from build123d import *

# Parameters (mm, degrees)
SKETCH1_W           = 12
SKETCH1_H           = 64.5
BOSS_EXTRUDE1_DEPTH = 5
FILLET1_R           = 6
SKETCH2_R           = 2
CUT_EXTRUDE1_DEPTH  = 34.182261828
BOSS_EXTRUDE2_START = 5
SKETCH3_R           = 6
SKETCH3_R_2         = 2
BOSS_EXTRUDE2_DEPTH = 5
SKETCH4_R           = 2
CUT_EXTRUDE2_DEPTH  = 34.182261828
CUT_EXTRUDE3_DEPTH  = 2.5


with BuildPart() as part:
    # Sketch1 → Boss-Extrude1 (new body)
    with BuildSketch(Plane(origin=(0, 0, 0), x_dir=(1, 0, 0), z_dir=(0, 1, 0))):
        Rectangle(SKETCH1_W, SKETCH1_H)
    extrude(amount=BOSS_EXTRUDE1_DEPTH)

    # Fillet1
    fillet1_edges = [part.edges().sort_by_distance(p)[0] for p in [
        (-6, 2.5, -32.25),
        (6, 2.5, -32.25),
        (-6, 2.5, 32.25),
        (6, 2.5, 32.25),
    ]]
    fillet(fillet1_edges, radius=FILLET1_R - 0.0001)  # a hair under: the kernel refuses the full size

    # Sketch2 → Cut-Extrude1 (cut, through all)
    with BuildSketch(Plane(origin=(0, 5, 0), x_dir=(1, 0, 0), z_dir=(0, 1, 0))):
        with Locations(Location((0, -26.25, 0), (0, 0, 270))):
            Circle(SKETCH2_R)
        with Locations(Location((0, 26.25, 0), (0, 0, 270))):
            Circle(SKETCH2_R)
    extrude(amount=-CUT_EXTRUDE1_DEPTH, mode=Mode.SUBTRACT)

    # Sketch3 → Boss-Extrude2 (add)
    # profile 1 of 2: a face of its own
    with BuildSketch(Plane(origin=(0, 5, 0), x_dir=(1, 0, 0), z_dir=(0, 1, 0)).offset(BOSS_EXTRUDE2_START)):
        with Locations(Location((0, -26.25, 0), (0, 0, 270))):
            Circle(SKETCH3_R)
        with Locations(Location((0, -26.25, 0), (0, 0, 270))):
            Circle(SKETCH3_R_2, mode=Mode.SUBTRACT)
    # profile 2 of 2: a face of its own
    with BuildSketch(Plane(origin=(0, 5, 0), x_dir=(1, 0, 0), z_dir=(0, 1, 0)).offset(BOSS_EXTRUDE2_START)):
        with Locations(Location((0, 26.25, 0), (0, 0, 90))):
            Circle(SKETCH3_R)
        with Locations(Location((0, 26.25, 0), (0, 0, 270))):
            Circle(SKETCH3_R_2, mode=Mode.SUBTRACT)
    extrude(amount=-BOSS_EXTRUDE2_DEPTH)

    # Sketch4 → Cut-Extrude2 (cut, through all)
    with BuildSketch(Plane(origin=(0, 5, 0), x_dir=(1, 0, 0), z_dir=(0, 1, 0))):
        with Locations(Location((0, 15, 0), (0, 0, 270))):
            Circle(SKETCH4_R)
        with Locations(Location((0, -15, 0), (0, 0, 270))):
            Circle(SKETCH4_R)
    extrude(amount=-CUT_EXTRUDE2_DEPTH, mode=Mode.SUBTRACT)

    # Sketch5 → Cut-Extrude3 (cut)
    with BuildSketch(Plane.XZ):
        Polygon((4.618802154, 26.25), (2.309401077, 30.25), (-2.309401077, 30.25), (-4.618802154, 26.25), (-2.309401077, 22.25), (2.309401077, 22.25), align=None)
        Polygon((2.309401077, -22.25), (-2.309401077, -22.25), (-4.618802154, -26.25), (-2.309401077, -30.25), (2.309401077, -30.25), (4.618802154, -26.25), align=None)
    extrude(amount=-CUT_EXTRUDE3_DEPTH, mode=Mode.SUBTRACT)


solid = part.part
For this review, take the finished solid that the model builds, in its own axes (mm). A direction names the side the tool comes from. Give positions to 0.01 mm unless a question says otherwise; leave off trailing zeros. Order: outer loops, then holes, each group sorted by start corner. A loop starts at its lowest first (then second) coordinate and runs counter-clockwise, first axis right, second up. Notation, with made-up numbers: M 65.5,57.25 L 92.5,57.25 A17 ccw 92.5,74.25 Z; hole C -4,78 d9. An arc over 180 degrees is marked long. Answer in a Markdown table with one row per item. Add a question column.
(1) Consider section C-C on y = 7.5. State the section outline as (x, z) points.
(2) For faces 5 (the face through (0, 1, 22.25)), 6 (the face through (-0.264, 7.535, -20.256)), 7 (the face through (0, 10, 29)), list the 3-axis set-ups (+Z, -Z, +X, -X, +Y, -Y) from which the entire face can be reached by the end or side of a thin tool; tool diameter is ignored.
(3) Consider section A-A on z = -15. State the section outline as (x, y) points.
(4) Consider section B-B on x = -1.25. Give the number of separate pieces and of enclosed holes in the cut face, and give its area (3 significant figures).
(5) Consider section D-D on z = -7.5. State the section outline as (x, y) points.
(6) For pin 1 (3 mm diameter, centred on x = 1, z = 2, fed in from +Y); pin 2 (2.5 mm diameter, centred on x = -1.5, z = -27.5, fed in from -Y); pin 3 (3.5 mm diameter, centred on x = 0, z = -15, fed in from +Y); pin 4 (6 mm diameter, centred on x = 4.5, y = 7.5, fed in from -Z), all flat-tipped, find the tip position at first contact; note any pin that passes through.
(7) Wall thickness on probe 1 along Z at (x, y) = (1.75, 7.25); probe 2 along X at (y, z) = (1, 15); probe 3 along X at (y, z) = (9.5, 28): over which ranges is each line inside the solid? List them lowest first. Write a range as [from, to].
(8) Mouldability with a two-part tool opening along Z and no side actions: class faces 1 (the face through (-4.289, 2.535, -30.446)), 2 (the face through (-4.289, 2.535, 30.446)), 3 (the face through (0, 1, -22.25)), 4 (the face through (0, 0, 0)) as +Z half, -Z half, draft (parallel to the pull), parting line (faces both ways), or undercut.
Evaluation:
| question | item | result |
|---|---|---|
| 1 | outline | C 0,-26.25 d12; C 0,26.25 d12; hole C 0,-26.25 d4; hole C 0,26.25 d4 |
| 2 | face 5 | -Y |
| 2 | face 6 | +Y |
| 2 | face 7 | +Z, -Z, +X, -X, +Y |
| 3 | outline | M -6,0 L -2,0 L -2,5 L -6,5 Z; M 2,0 L 6,0 L 6,5 L 2,5 Z |
| 4 | separate pieces | 5 |
| 4 | enclosed holes | 0 |
| 4 | area | 320 mm^2 |
| 5 | outline | M -6,0 L 6,0 L 6,5 L -6,5 Z |
| 6 | pin 1 | stops at y = 5 |
| 6 | pin 2 | stops at y = 2.5 |
| 6 | pin 3 | passes through |
| 6 | pin 4 | stops at z = -32.06 |
| 7 | probe 1 | z = [-31.99, -27.22], [-25.28, -20.51], [20.51, 25.28], [27.22, 31.99] |
| 7 | probe 2 | x = [-6, -2], [2, 6] |
| 7 | probe 3 | x = [-5.74, -0.97], [0.97, 5.74] |
| 8 | face 1 | -Z half |
| 8 | face 2 | +Z half |
| 8 | face 3 | undercut |
| 8 | face 4 | draft |
